The listing builds one solid part. Answer for the finished solid, in the listing's coordinates (mm). Give positions to 0.01 mm unless a question says otherwise; leave off trailing zeros. Write each loop counter-clockwise with the first axis right and the second up, starting at its lowest first coordinate (ties: lowest second). Pieces come first, ordered by that corner, then holes. Notation, with made-up numbers: (81.5, 9.25) -> (102.5, 9.25) arc R24 cw to (102.5, 47.25) -> close; hole circle Ø6 at (58, 29). An arc over 180 degrees is marked (long way). Put each result on its own line as item: value. Start each with the question number.
1) For a pull along Y with two mould halves and no side action, classify faces 1 (the flat face through (3.944, -12.805, -12.537)), 2 (the flat face through (3.944, 7.966, -16.053)), 3 (the cylindrical face through (3.94, -29.97, 1.32)) as released by +Y, released by -Y, zero draft, split by the parting line, or undercut.
2) A cutting plane is placed at A-A (z = 15). Write down the section's boundary in (x, y).
3) A cutting plane is placed at B-B (y = -16.5). Write down the section's boundary in (x, z), then the cut area to 3 significant figures.
4) A cutting plane is placed at C-C (x = 6.5). Give the number of separate pieces and of enclosed holes in the cut face, then the cut area to 3 significant figures.
5) Flat-ended cylindrical pins translate along their axes: pin 1 Ø1 at (x, z) = (6.5, 9) entering from -Y; pin 2 Ø1.8 at (y, z) = (6.35, 0) entering from +X; pin 3 Ø1 at (x, z) = (4.5, -18) entering from +Y; pin 4 Ø1.5 at (x, y) = (4.5, 0) entering from +Z. Find the tip coordinate at first contact, or state that the pin passes through.
6) Find the intervals of material crossed by line 1 along Z through (x, y) = (6.25, 6.35); line 2 along Z through (x, y) = (4, -22); line 3 along Y through (x, z) = (7.5, 17), in increasing order. Write a range as from..to.
from build123d import *

# Parameters (mm, degrees)
F0_R     = 29.99994
F0_R_2   = 1.1303
F1_DEPTH = 8.000009


with BuildPart() as f1:
    # F0 (on Right) → F1 (new body)
    with BuildSketch(Plane.YZ):
        Circle(F0_R)
        with BuildLine():
            Line((-13.640059, -23.095236), (-2.449158, -9.204741))
            ThreePointArc((-2.449158, -9.204741), (0, -9.525), (2.449158, -9.204741))
            Line((2.449158, -9.204741), (13.640059, -23.095236))
            ThreePointArc((13.640059, -23.095236), (0, -26.8224), (-13.640059, -23.095236))
        make_face(mode=Mode.SUBTRACT)
        with BuildLine():
            Line((-26.179885, 5.835646), (-9.51106, -0.515133))
            ThreePointArc((-9.51106, -0.515133), (-9.058813, -2.943387), (-7.997397, -5.173709))
            Line((-7.997397, -5.173709), (-17.749865, -20.109287))
            ThreePointArc((-17.749865, -20.109287), (-25.509618, -8.288577), (-26.179885, 5.835646))
        make_face(mode=Mode.SUBTRACT)
        with BuildLine():
            ThreePointArc((-6.05216, -9.489048), (-5.897812, -9.781454), (-5.973962, -10.103209))
            ThreePointArc((-5.973962, -10.103209), (-5.98861, -10.123802), (-6.004343, -10.143579))
            Line((-6.004343, -10.143579), (-13.850079, -20.568703))
            ThreePointArc((-13.850079, -20.568703), (-14.017097, -20.66058), (-14.203454, -20.620481))
            Line((-14.203454, -20.620481), (-15.222134, -19.880366))
            ThreePointArc((-15.222134, -19.880366), (-15.317858, -19.715522), (-15.282089, -19.528287))
            Line((-15.282089, -19.528287), (-7.791673, -8.845008))
            ThreePointArc((-7.791673, -8.845008), (-7.777726, -8.823934), (-7.762667, -8.803639))
            ThreePointArc((-7.762667, -8.803639), (-7.480192, -8.631788), (-7.1544, -8.688223))
            Line((-7.1544, -8.688223), (-6.05216, -9.489048))
        make_face(mode=Mode.SUBTRACT)
        with BuildLine():
            ThreePointArc((7.1544, -8.688223), (7.480192, -8.631788), (7.762667, -8.803639))
            ThreePointArc((7.762667, -8.803639), (7.777726, -8.823934), (7.791673, -8.845008))
            Line((7.791673, -8.845008), (15.282089, -19.528287))
            ThreePointArc((15.282089, -19.528287), (15.317858, -19.715522), (15.222134, -19.880366))
            Line((15.222134, -19.880366), (14.203454, -20.620481))
            ThreePointArc((14.203454, -20.620481), (14.017097, -20.66058), (13.850079, -20.568703))
            Line((13.850079, -20.568703), (6.004343, -10.143579))
            ThreePointArc((6.004343, -10.143579), (5.98861, -10.123802), (5.973962, -10.103209))
            ThreePointArc((5.973962, -10.103209), (5.897812, -9.781454), (6.05216, -9.489048))
            Line((6.05216, -9.489048), (7.1544, -8.688223))
        make_face(mode=Mode.SUBTRACT)
        with BuildLine():
            ThreePointArc((1.32334, 1.508382), (0, -2.0066), (-1.32334, 1.508382))
            Line((-1.32334, 1.508382), (1.32334, 1.508382))
        make_face(mode=Mode.SUBTRACT)
        with BuildLine():
            Line((17.749865, -20.109287), (7.997397, -5.173709))
            ThreePointArc((7.997397, -5.173709), (9.058813, -2.943387), (9.51106, -0.515133))
            Line((9.51106, -0.515133), (26.179885, 5.835646))
            ThreePointArc((26.179885, 5.835646), (25.509618, -8.288577), (17.749865, -20.109287))
        make_face(mode=Mode.SUBTRACT)
        with BuildLine():
            ThreePointArc((-10.894841, 2.823669), (-11.12524, 2.586517), (-11.454779, 2.559512))
            ThreePointArc((-11.454779, 2.559512), (-11.478891, 2.56708), (-11.502561, 2.575932))
            Line((-11.502561, 2.575932), (-23.841909, 6.816129))
            ThreePointArc((-23.841909, 6.816129), (-23.980901, 6.946581), (-24.000351, 7.136208))
            Line((-24.000351, 7.136208), (-23.61125, 8.333739))
            ThreePointArc((-23.61125, 8.333739), (-23.484054, 8.475717), (-23.294929, 8.499558))
            Line((-23.294929, 8.499558), (-10.819862, 4.677063))
            ThreePointArc((-10.819862, 4.677063), (-10.795509, 4.670311), (-10.771554, 4.662261))
            ThreePointArc((-10.771554, 4.662261), (-10.520825, 4.446716), (-10.473823, 4.11943))
            Line((-10.473823, 4.11943), (-10.894841, 2.823669))
        make_face(mode=Mode.SUBTRACT)
        with Locations((-6.35, 0)):
            Circle(F0_R_2, mode=Mode.SUBTRACT)
        with BuildLine():
            ThreePointArc((-24.610079, 10.667013), (-15.765811, 21.699777), (-2.54, 26.701864))
            Line((-2.54, 26.701864), (-3.429, 8.886371))
            ThreePointArc((-3.429, 8.886371), (-5.598655, 7.705887), (-7.391821, 6.007212))
            Line((-7.391821, 6.007212), (-24.610079, 10.667013))
        make_face(mode=Mode.SUBTRACT)
        with Locations((6.35, 0)):
            Circle(F0_R_2, mode=Mode.SUBTRACT)
        with BuildLine():
            ThreePointArc((10.473823, 4.11943), (10.520825, 4.446716), (10.771554, 4.662261))
            ThreePointArc((10.771554, 4.662261), (10.795509, 4.670311), (10.819862, 4.677063))
            Line((10.819862, 4.677063), (23.294929, 8.499558))
            ThreePointArc((23.294929, 8.499558), (23.484054, 8.475717), (23.61125, 8.333739))
            Line((23.61125, 8.333739), (24.000351, 7.136208))
            ThreePointArc((24.000351, 7.136208), (23.980901, 6.946581), (23.841909, 6.816129))
            Line((23.841909, 6.816129), (11.502561, 2.575932))
            ThreePointArc((11.502561, 2.575932), (11.478891, 2.56708), (11.454779, 2.559512))
            ThreePointArc((11.454779, 2.559512), (11.12524, 2.586517), (10.894841, 2.823669))
            Line((10.894841, 2.823669), (10.473823, 4.11943))
        make_face(mode=Mode.SUBTRACT)
        with BuildLine():
            Line((0.681222, 11.234171), (-0.681222, 11.234171))
            ThreePointArc((-0.681222, 11.234171), (-0.977964, 11.38001), (-1.105481, 11.685075))
            ThreePointArc((-1.105481, 11.685075), (-1.105734, 11.710345), (-1.10463, 11.735592))
            Line((-1.10463, 11.735592), (-0.885031, 24.781302))
            ThreePointArc((-0.885031, 24.781302), (-0.803914, 24.953804), (-0.629579, 25.0309))
            Line((-0.629579, 25.0309), (0.629579, 25.0309))
            ThreePointArc((0.629579, 25.0309), (0.803914, 24.953804), (0.885031, 24.781302))
            Line((0.885031, 24.781302), (1.10463, 11.735592))
            ThreePointArc((1.10463, 11.735592), (1.105734, 11.710345), (1.105481, 11.685075))
            ThreePointArc((1.105481, 11.685075), (0.977964, 11.38001), (0.681222, 11.234171))
        make_face(mode=Mode.SUBTRACT)
        with BuildLine():
            Line((3.429, 8.886371), (2.54, 26.701864))
            ThreePointArc((2.54, 26.701864), (15.765811, 21.699777), (24.610079, 10.667013))
            Line((24.610079, 10.667013), (7.391821, 6.007212))
            ThreePointArc((7.391821, 6.007212), (5.598655, 7.705887), (3.429, 8.886371))
        make_face(mode=Mode.SUBTRACT)
    extrude(amount=F1_DEPTH)


solid = f1.part
Reply:
1. face 1: undercut
1. face 2: undercut
1. face 3: split by the parting line
2. outline: (0, -25.98) -> (8, -25.98) -> (8, -22.24) -> (0, -22.24) -> close; (0, -3.12) -> (8, -3.12) -> (8, -1.05) -> (0, -1.05) -> close; (0, 1.05) -> (8, 1.05) -> (8, 3.12) -> (0, 3.12) -> close; (0, 22.24) -> (8, 22.24) -> (8, 25.98) -> (0, 25.98) -> close
3. outline: (0, -25.05) -> (8, -25.05) -> (8, -18.2) -> (0, -18.2) -> close; (0, 2.15) -> (8, 2.15) -> (8, 4.29) -> (0, 4.29) -> close; (0, 6.42) -> (8, 6.42) -> (8, 8.47) -> (0, 8.47) -> close; (0, 21.15) -> (8, 21.15) -> (8, 25.05) -> (0, 25.05) -> close
3. area: 120 mm2
4. separate pieces: 1
4. enclosed holes: 13
4. area: 1,210 mm2
5. pin 1: stops at y = -28.77
5. pin 2: passes through
5. pin 3: stops at y = 24.37
5. pin 4: stops at z = 30
6. line 1: z = -29.32..-26.06, -14.05..-10.6, -9.27..-1.13, 1.13..7.1, 26.06..29.32
6. line 2: z = -20.4..-15.34, 4.24..6.18, 8.1..9.96, 15.34..20.4
6. line 3: y = -24.72..-20.75, -3.02..-1.02, 1.02..3.02, 20.75..24.72
